The listing builds one solid part. Answer for the finished solid, in the listing's coordinates (mm). Round coordinates to 2 decimals unless told otherwise and drop trailing zeros. Answer as a JSON object with one key per item and string values.
```python
from build123d import *

# Parameters (mm, degrees)
SKETCH_1_W          = 1600
SKETCH_1_H          = 1230
SKETCH_1_R          = 15
EXTRUDE_1_DEPTH     = 3
SCALE_1_SCALE_X     = 0.1
SCALE_1_SCALE_Y     = 0.1
SCALE_1_SCALE_Z     = 0.5
SKETCH_2_W          = 29.5
SKETCH_2_H          = 63.1
CUT_EXTRUDE_1_DEPTH = 2.5000001


with BuildPart() as part:
    # 草图1 → 凸台-拉伸1 (new body)
    with BuildSketch(Plane.XY):
        with Locations((1152.60835314, -1687.80288964)):
            Rectangle(SKETCH_1_W, SKETCH_1_H)
        with Locations((417.60835314, -1137.80288964)):
            Circle(SKETCH_1_R, mode=Mode.SUBTRACT)
        with Locations((1887.60835314, -1137.80288964)):
            Circle(SKETCH_1_R, mode=Mode.SUBTRACT)
        with Locations((1887.60835314, -2237.80288964)):
            Circle(SKETCH_1_R, mode=Mode.SUBTRACT)
        with Locations((417.60835314, -2237.80288964)):
            Circle(SKETCH_1_R, mode=Mode.SUBTRACT)
    extrude(amount=EXTRUDE_1_DEPTH)


with BuildPart() as part_1:
    # 缩放比例1: scaled about (1152.60835314, -1687.80288964, 1.5)
    add(part.part.scale((SCALE_1_SCALE_X, SCALE_1_SCALE_Y, SCALE_1_SCALE_Z), about=(1152.60835314, -1687.80288964, 1.5)))

    # 草图2 → 切除-拉伸1 (cut, through all)
    with BuildSketch(Plane.XY.offset(2.25)):
        with Locations((1087.35835314, -1702.21288964)):
            Rectangle(SKETCH_2_W, SKETCH_2_H)
    extrude(amount=-CUT_EXTRUDE_1_DEPTH, mode=Mode.SUBTRACT)


solid = part_1.part
```
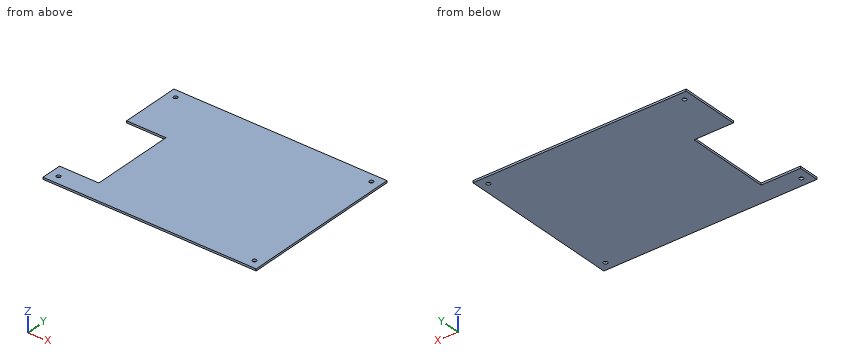
Item 1: A flat-ended cylindrical pin translates along its axis: P1, Ø0.8, axis at y = -1704.5, z = 1.5, coming from the -X side. Find the tip coordinate at first contact, or state that the pin passes through.
Values follow:
{"P1": "x = 1102.11"}
Item 2: The part is cut by section A-A (z = 1.85). Give the number of separate pieces and of enclosed holes in the cut face, then the cut area to 3 significant figures.
Values follow:
{"separate pieces": "1", "enclosed holes": "4", "area": "17,800 mm^2"}
Item 3: Straight lines are drawn through the part: line 1 (Y direction, x = 1097, z = 1.3); line 2 (X direction, y = -1730.5, z = 1.1). For each, find the intervals that lie inside material, in ascending order.
Values follow:
{"line 1": "-1749.3 to -1733.76, -1670.66 to -1626.3", "line 2": "1102.11 to 1232.61"}
